```python
from build123d import *
from build123d.topology import SkipClean

# Parameters (mm, degrees)
SKETCH1_R                                       = 3.175
EXTRUDE_BODY_DEPTH                              = 5
INSET_BODY_DEPTH                                = 2
SKETCH3_R                                       = 6.175
CUT_HOLE_BOSS_DEPTH                             = 5
CUT_EXTRUDE2_DEPTH                              = 72.874270106
CUT_EXTRUDE2_DEPTH_BACK                         = 5
REAM_HOLE_R                                     = 3.175
SKETCH4_W                                       = 32.629490944
SKETCH4_H                                       = 4.242640687
BOSS_EXTRUDE1_DEPTH                             = 15
CSK_FOR_M3_FLAT_HEAD_MACHINE_SCREW1_D           = 3.4
CSK_FOR_M3_FLAT_HEAD_MACHINE_SCREW1_CSINK_D     = 6.3
CSK_FOR_M3_FLAT_HEAD_MACHINE_SCREW1_CSINK_ANGLE = 90


with BuildPart() as part:
    # Sketch1 → Extrude body (new body)
    with BuildSketch(Plane(origin=(0, 0, 0), x_dir=(0, 0, -1), z_dir=(1, 0, 0))):
        with BuildLine():
            Line((8.114294626, 0), (-24.515196318, 0))
            Line((-24.515196318, 0), (-24.515196318, 24.898772612))
            ThreePointArc((-24.515196318, 24.898772612), (-21.586264129, 31.969840424), (-14.515196318, 34.898772612))
            Line((-14.515196318, 34.898772612), (5.191949728, 34.898772612))
            ThreePointArc((5.191949728, 34.898772612), (9.018784051, 35.659977287), (12.26301754, 37.8277048))
            Line((12.26301754, 37.8277048), (26.380592117, 51.945279378))
            ThreePointArc((26.380592117, 51.945279378), (33.451659929, 54.874211566), (40.52272774, 51.945279378))
            Line((40.52272774, 51.945279378), (43.22008306, 49.247924058))
            ThreePointArc((43.22008306, 49.247924058), (46.149015248, 42.176856246), (43.22008306, 35.105788434))
            Line((43.22008306, 35.105788434), (8.114294626, 0))
        make_face()
        with Locations((31.264803682, 39.99)):
            Circle(SKETCH1_R, mode=Mode.SUBTRACT)
        with Locations((-9.515196318, 19.93)):
            Circle(SKETCH1_R, mode=Mode.SUBTRACT)
    extrude(amount=EXTRUDE_BODY_DEPTH)

    # Sketch2 → Inset body (cut)
    with BuildSketch(Plane(origin=(0, 0, 0), x_dir=(0, 0, -1), z_dir=(1, 0, 0))):
        with BuildLine():
            Line((-21.515196318, 24.898772612), (-21.515196318, 3))
            Line((-21.515196318, 3), (6.871653938, 3))
            Line((6.871653938, 3), (41.098762716, 37.227108778))
            ThreePointArc((41.098762716, 37.227108778), (43.149015248, 42.176856246), (41.098762716, 47.126603714))
            Line((41.098762716, 47.126603714), (38.401407397, 49.823959034))
            ThreePointArc((38.401407397, 49.823959034), (33.451659929, 51.874211566), (28.50191246, 49.823959034))
            Line((28.50191246, 49.823959034), (14.384337883, 35.706384457))
            ThreePointArc((14.384337883, 35.706384457), (10.166834349, 32.88833869), (5.191949728, 31.898772612))
            Line((5.191949728, 31.898772612), (-14.515196318, 31.898772612))
            ThreePointArc((-14.515196318, 31.898772612), (-19.464943786, 29.848520081), (-21.515196318, 24.898772612))
        make_face()
    extrude(amount=INSET_BODY_DEPTH, mode=Mode.SUBTRACT)

    # Sketch3 → Cut hole boss (add)
    with BuildSketch(Plane.ZY.offset(-2)):
        with Locations(Location((9.515196318, 19.93, 0), (0, 0, 180))):
            Circle(SKETCH3_R)
        with Locations(Location((-31.264803682, 39.99, 0), (0, 0, 180))):
            Circle(SKETCH3_R)
    extrude(amount=CUT_HOLE_BOSS_DEPTH)

    # Ream hole → Cut-Extrude2 (cut, two sides: drawn at the far end of the back side and taken through both)
    with SkipClean():  # the faces are left unmerged after this step: merging them gives an invalid solid
        with BuildSketch(Plane.ZY.offset(-CUT_EXTRUDE2_DEPTH_BACK)):
            with Locations((-31.264803682, 39.99)):
                Circle(REAM_HOLE_R)
            with Locations((9.515196318, 19.93)):
                Circle(REAM_HOLE_R)
        extrude(amount=CUT_EXTRUDE2_DEPTH + CUT_EXTRUDE2_DEPTH_BACK, mode=Mode.SUBTRACT)

    # Sketch4 → Boss-Extrude1 (add)
    with SkipClean():  # the faces are left unmerged after this step: merging them gives an invalid solid
        with BuildSketch(Plane.ZY.offset(-2)):
            with Locations((8.200450846, 2.121320344)):
                Rectangle(SKETCH4_W, SKETCH4_H)
        extrude(amount=BOSS_EXTRUDE1_DEPTH)

    # CSK for M3 Flat Head Machine Screw1 (through all)
    with Locations(Plane(origin=(0, 4.242640687, 0), x_dir=(1, 0, 0), z_dir=(0, 1, 0))):
        with Locations((-6.5, -8.200450846)):
            CounterSinkHole(CSK_FOR_M3_FLAT_HEAD_MACHINE_SCREW1_D / 2, CSK_FOR_M3_FLAT_HEAD_MACHINE_SCREW1_CSINK_D / 2, counter_sink_angle=CSK_FOR_M3_FLAT_HEAD_MACHINE_SCREW1_CSINK_ANGLE)


solid = part.part
```
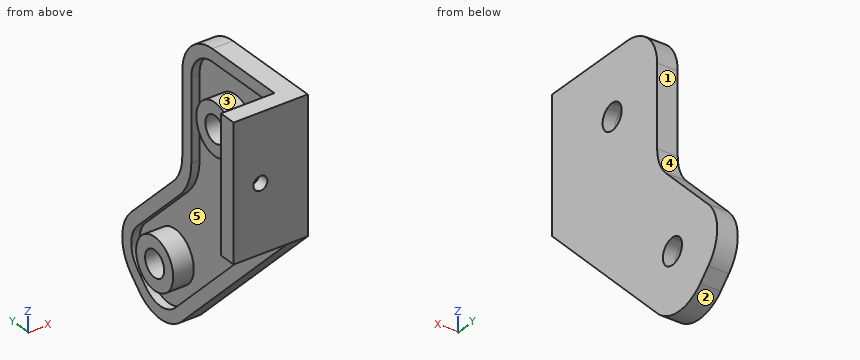
Input: part model. Units: mm. Frame: model coordinates. Face numbers are marked on the shaded views. A direction names the side the tool comes from. Coordinates: 2 decimals unless noted, no trailing zeros. Loops run counter-clockwise (first coordinate to the right, second up) from the corner with the lowest first, then second, coordinate; pieces in that order, holes last.
Q1. Set-up query: the marked faces 4 and 5. Return all of +Z, -Z, +X, -X, +Y, -Y with unobstructed straight access to the full face (end or side cutting, diameter ignored); none if empty.
Results are:
face 4: +Z, +X, -X, +Y
face 5: -X
Q2. Section A-A, the plane x = -6.5. Return the cut outline in (y, z), and give its area (3 significant figures).
Results are:
outline: (0, -8.11) - (4.24, -8.11) - (4.24, 5.05) - (2.79, 6.5) - (0, 6.5) - close; (0, 9.9) - (2.79, 9.9) - (4.24, 11.35) - (4.24, 24.52) - (0, 24.52) - close
area: 122 mm2
Q3. Section C-C, the plane y = 12.5. Return the cut outline in (x, z).
Results are:
outline: (0, -20.61) - (5, -20.61) - (5, 24.52) - (0, 24.52) - (0, 21.52) - (2, 21.52) - (2, -16.37) - (0, -16.37) - close
Q4. Mould query, pull axis Y, two halves, no side actions, for the marked faces 1, 2 and 3. Classes: +Y half, -Y half, draft (parallel to the pull), parting line (faces both ways), or undercut.
Results are:
face 1: +Y half
face 2: parting line
face 3: undercut
Q5. Section B-B, the plane z = -10.5. Return the cut outline in (x, y), and give its area (3 significant figures).
Results are:
outline: (0, 2.39) - (5, 2.39) - (5, 36.42) - (0, 36.42) - (0, 33.03) - (2, 33.03) - (2, 6.63) - (0, 6.63) - close
area: 117 mm2
Q6. Contact query for flat-ended pins moving along their axis: pin 1 (24 mm diameter, centred on y = 35, z = -17, fed in from -X); pin 2 (1.3 mm diameter, centred on x = -9.5, y = 2, fed in from -Z); pin 3 (1 mm diameter, centred on x = 1, y = 15, fed in from -Z). Output: stop coordinate, or through.
Results are:
pin 1: stops at x = -3
pin 2: stops at z = -8.11
pin 3: stops at z = -23.61
Q7. Line query: line 1 along Z through (x, y) = (-2, 19.93); line 2 along Z through (x, y) = (-1.1, 39.99); line 3 along Z through (x, y) = (0.5, 17.5). Output: solid intervals per line, ascending.
Results are:
line 1: z = 3.34 to 6.34, 12.69 to 15.69
line 2: z = -37.44 to -34.44, -28.09 to -25.09
line 3: z = -25.61 to -21.37, 3.84 to 7.47, 11.56 to 15.19, 21.52 to 24.52
Q8. Section D-D, the plane z = -36. Return the cut outline in (x, y).
Results are:
outline: (-3, 36.03) - (2, 36.03) - (2, 32.13) - (0, 32.13) - (0, 27.89) - (5, 27.89) - (5, 54.54) - (0, 54.54) - (0, 51.39) - (2, 51.39) - (2, 43.95) - (-3, 43.95) - close
